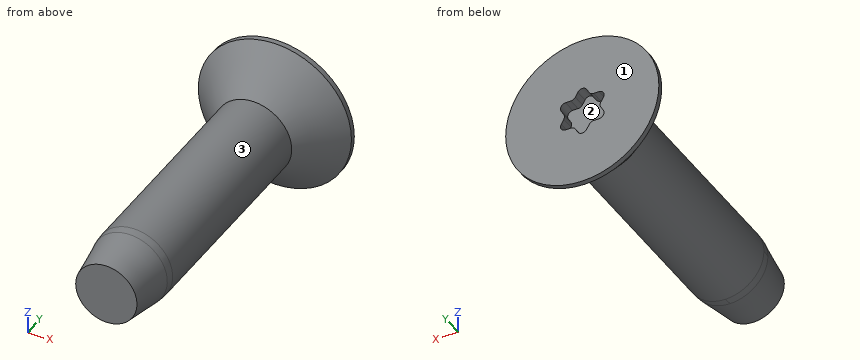
```python
from build123d import *

# Parameters (mm, degrees)
SKETCH2_R           = 1.5
BOSS_EXTRUDE1_DEPTH = 10.3
CUT_EXTRUDE1_DEPTH  = 0.5
FILLET1_R           = 0.2
FILLET3_R           = 2


with BuildPart() as part:
    # Sketch1 → Revolve1 (revolve)
    with BuildSketch(Plane.XY, mode=Mode.PRIVATE) as revolve1_sk:
        Polygon((0, 0), (0, 1.7), (3, 1.7), (3, 1.5), (1.5, 0), align=None)
    revolve(revolve1_sk.sketch.rotate(Axis((0, 50, 0), (0, -1, 0)), 90), axis=Axis((0, 50, 0), (0, -1, 0)))

    # Sketch2 → Boss-Extrude1 (add)
    with BuildSketch(Plane.XZ):
        with Locations(Location((0, 0, 0), (0, 0, 270))):
            Circle(SKETCH2_R)
    extrude(amount=BOSS_EXTRUDE1_DEPTH)

    # Sketch3 → Cut-Revolve1 (revolve, cut)
    with BuildSketch(Plane.XY, mode=Mode.PRIVATE) as cut_revolve1_sk:
        Polygon((1.5, -8.5), (1.2, -10.3), (1.5, -10.3), align=None)
    revolve(cut_revolve1_sk.sketch.rotate(Axis((0, 0, 0), (0, -1, 0)), 180), axis=Axis((0, 0, 0), (0, -1, 0)), mode=Mode.SUBTRACT)

    # Sketch4 → Cut-Extrude1 (cut)
    with BuildSketch(Plane(origin=(0, 1.7, 0), x_dir=(1, 0, 0), z_dir=(0, 1, 0))):
        Polygon((0, 1.152050808), (0.330273688, 0.58), (1, 0.58), (0.665136844, 0), (1, -0.58), (0.330273688, -0.58), (0, -1.152050808), (-0.330273688, -0.58), (-1, -0.58), (-0.665136844, 0), (-1, 0.58), (-0.330273688, 0.58), align=None)
    extrude(amount=-CUT_EXTRUDE1_DEPTH, mode=Mode.SUBTRACT)

    # Fillet1
    fillet1_edges = [part.edges().sort_by_distance(p)[0] for p in [
        (-0.330273688, 1.45, -0.58),
        (0, 1.45, -1.152050808),
        (0.330273688, 1.45, -0.58),
        (1, 1.45, -0.58),
        (0.665136844, 1.45, 0),
        (1, 1.45, 0.58),
        (0.330273688, 1.45, 0.58),
        (0, 1.45, 1.152050808),
        (-0.330273688, 1.45, 0.58),
        (-1, 1.45, 0.58),
        (-0.665136844, 1.45, 0),
        (-1, 1.45, -0.58),
    ]]
    fillet(fillet1_edges, radius=FILLET1_R)

    # Fillet3
    fillet3_edges = [part.edges().sort_by_distance(p)[0] for p in [
        (-1.060660172, -8.5, -1.060660172),
    ]]
    fillet(fillet3_edges, radius=FILLET3_R)


solid = part.part
```
The model under review builds one solid part; all positions refer to its coordinate system, in mm. Face numbers are marked on the shaded views. Give positions to 0.01 mm unless a question says otherwise; leave off trailing zeros. Write each loop counter-clockwise with the first axis right and the second up, starting at its lowest first coordinate (ties: lowest second). Pieces come first, ordered by that corner, then holes. Notation, with made-up numbers: M 18.5,12 L 26.5,12 A18 ccw 26.5,35 Z; hole C 77,5 d1. An arc over 180 degrees is marked long. Answer in a Markdown table with one row per item.
Item 1: For line 1 along Y through (x, z) = (-0.5, 0.45); line 2 along X through (y, z) = (-0.75, 0.1); line 3 along Y through (x, z) = (2.2, -0.75), list the stretches that pass through material, from the lowest coordinate up.
Check sheet entries:
| item | result |
|---|---|
| line 1 | -10.3 to 1.2 |
| line 2 | -1.5 to 1.5 |
| line 3 | 0.82 to 1.7 |
Item 2: Add section B-B on y = -5. Give the boundary of the cut face in (x, z), plus the area to 3 significant figures.
Check sheet entries:
| item | result |
|---|---|
| outline | C 0,0 d3 |
| area | 7.07 mm2 |
Item 3: Draft analysis for pull direction X (two halves, no side actions). For the marked faces 1, 2 and 3, state which applies: +X half, -X half, draft (parallel to the pull), parting line (faces both ways), or undercut.
Check sheet entries:
| item | result |
|---|---|
| face 1 | draft |
| face 2 | undercut |
| face 3 | parting line |
Item 4: For P1, Ø2, axis at x = 0.5, y = -3, coming from the +Z side; P2, Ø1.5, axis at y = -0.5, z = -1, coming from the -X side; P3, Ø1.9, axis at x = 0.5, z = -0.5, coming from the +Y side; P4, Ø1, axis at x = -0.5, y = -6.5, coming from the -Z side, all flat-tipped, find the tip position at first contact; note any pin that passes through.
Check sheet entries:
| item | result |
|---|---|
| P1 | z = 1.5 |
| P2 | x = -1.54 |
| P3 | y = 1.7 |
| P4 | z = -1.5 |
Item 5: Add section A-A on y = 1. Give the boundary of the cut face in (x, z).
Check sheet entries:
| item | result |
|---|---|
| outline | C 0,0 d5 |
